Geometry check sheet. Reference: the model listing, model coordinates, mm. Face numbers are marked on the shaded views. A direction names the side the tool comes from. Give positions to 0.01 mm unless a question says otherwise; leave off trailing zeros. Order: outer loops, then holes, each group sorted by start corner. A loop starts at its lowest first (then second) coordinate and runs counter-clockwise, first axis right, second up. Notation, with made-up numbers: M -3,41.25 L 29,41.25 A10 cw 29,58.25 Z; hole C 17.5,73 d8. An arc over 180 degrees is marked long. Answer as CSV lines item,"result". Start each with the question number.
Q1. Go/stop test with flat-tipped pins: pin 1 (6 mm diameter, centred on x = 73.5, z = -8, fed in from -Y); pin 2 (3 mm diameter, centred on y = 19, z = -39.5, fed in from +X); pin 3 (6 mm diameter, centred on y = 28.5, z = -6.5, fed in from -X). Record where each tip stops, or that it passes through.
Q2. Section check C-C, the plane x = 60.5. Record the boundary of the cut face in (y, z) (3 decimals), then the cut area to 3 significant figures.
Q3. Set-up check for the marked faces 1 and 2: record each of +Z, -Z, +X, -X, +Y, -Y from which the full face is reachable in a straight line by a thin tool's end or side.
Q4. Section check B-B, the plane x = 25. Count the separate pieces of the cut face and the enclosed holes in it, then the cut area to 3 significant figures.
Q5. Thickness scan on line 1 (Y direction, x = 25, z = -40.5); line 2 (X direction, y = 10.75, z = -40); line 3 (Z direction, x = 37.5, y = 21.25). Record the ranges inside material, lowest first.
Q6. Mould release check, pull along Z, two halves, no side actions. Record for the marked faces 3, 4 and 5: +Z half, -Z half, draft (parallel to the pull), parting line (faces both ways), or undercut.
Q7. Section check A-A, the plane x = 80. Record the boundary of the cut face in (y, z) (3 decimals), then the cut area to 3 significant figures.
```python
from build123d import *

# Parameters (mm, degrees)
SKETCH_1_W               = 90
SKETCH_1_H               = 45
EXTRUDE_1_DEPTH          = 60
CUT_EXTRUDE_1_DEPTH      = 118.153745139
CUT_EXTRUDE_1_DEPTH_BACK = 118.153745139
CUT_EXTRUDE_2_DEPTH      = 105.446158378
EXTRUDE_3_REACH          = 105.804
SKETCH_4_W               = 86
SKETCH_4_H               = 41
SKETCH_4_W_2             = 82
SKETCH_4_H_2             = 34
CUT_EXTRUDE_3_DEPTH      = 105.522724802
SKETCH_6_W               = 72
SKETCH_6_H               = 33
CUT_EXTRUDE_4_DEPTH      = 98.541192544
EXTRUDE_8_DEPTH          = 82
CUT_EXTRUDE_5_REACH      = 99.614
SKETCH_10_W              = 79
SKETCH_10_H              = 27.766838789
SKETCH_11_W              = 3
SKETCH_11_H              = 42.766838789
CUT_EXTRUDE_6_DEPTH      = 5
EXTRUDE_9_DEPTH          = 28
SKETCH_13_R              = 1.5
CUT_EXTRUDE_7_DEPTH      = 104.169264805
FILLET_1_R               = 1
FILLET_2_R               = 1
FILLET_3_R               = 1
CUT_EXTRUDE_8_DEPTH      = 1


with BuildPart() as part:
    # 草图1 → 凸台-拉伸1 (new body)
    with BuildSketch(Plane(origin=(0, 0, 0), x_dir=(1, 0, 0), z_dir=(0, 1, 0))):
        with Locations((45, 22.5)):
            Rectangle(SKETCH_1_W, SKETCH_1_H)
    extrude(amount=EXTRUDE_1_DEPTH)

    # 草图2 → 切除-拉伸1 (cut, two sides: drawn at the far end of the back side and taken through both)
    with BuildSketch(Plane(origin=(90, 0, 0), x_dir=(0, 0, -1), z_dir=(1, 0, 0)).offset(-CUT_EXTRUDE_1_DEPTH_BACK)):
        Polygon((0, 220), (0, 60), (0, 28), (40, 10), (45, 10), (205, 10), (433.983745882, 233.531751932), (228.983745882, 443.531751932), align=None)
    extrude(amount=CUT_EXTRUDE_1_DEPTH + CUT_EXTRUDE_1_DEPTH_BACK, mode=Mode.SUBTRACT)

    # 草图3 → 切除-拉伸2 (cut, through all)
    with BuildSketch(Plane(origin=(90, 0, 0), x_dir=(0, 0, -1), z_dir=(1, 0, 0))):
        Polygon((0, 26.44865757), (39.885905712, 8.5), (45, 8.5), (45, 0), (0, 0), align=None)
    extrude(amount=-CUT_EXTRUDE_2_DEPTH, mode=Mode.SUBTRACT)

    # 草图4 → 凸台-拉伸3 (add, up to next)
    with BuildSketch(Plane(origin=(0, 34, 0), x_dir=(1, 0, 0), z_dir=(0, 1, 0)), mode=Mode.PRIVATE) as extrude_3_sk1:
        with Locations((45, 22.5)):
            Rectangle(SKETCH_4_W, SKETCH_4_H)
        with Locations((45, 21)):
            Rectangle(SKETCH_4_W_2, SKETCH_4_H_2, mode=Mode.SUBTRACT)
    extrude_3_tool1 = extrude(extrude_3_sk1.sketch, amount=-EXTRUDE_3_REACH, mode=Mode.PRIVATE) - part.part
    add(extrude_3_tool1.solids().sort_by_distance((45, 34, -2.952733))[0])

    # 草图5 → 切除-拉伸3 (cut, through all)
    with BuildSketch(Plane.ZY.offset(-2)):
        Polygon((-43, 15.03292805), (-41, 15.03292805), (-2, 32.58292805), (-2, 34), (-43, 34), align=None)
    extrude(amount=-CUT_EXTRUDE_3_DEPTH, mode=Mode.SUBTRACT)

    # 草图6 → 切除-拉伸4 (cut, through all)
    with BuildSketch(Plane(origin=(0, 21.99472563, -9.897626534), x_dir=(1, 0, 0), z_dir=(0, -0.9119215051751064, 0.41036467732879806))):
        with Locations((49, -11.015560293)):
            Rectangle(SKETCH_6_W, SKETCH_6_H)
    extrude(amount=-CUT_EXTRUDE_4_DEPTH, mode=Mode.SUBTRACT)

    # 草图9 → 凸台-拉伸8 (add)
    with BuildSketch(Plane(origin=(4, 0, 0), x_dir=(0, 0, -1), z_dir=(1, 0, 0))):
        Polygon((4, 31.68292805), (4, 30.58634244), (38, 15.28634244), (38, 16.38292805), align=None)
    extrude(amount=EXTRUDE_8_DEPTH)

    # 草图10 → 切除-拉伸5 (cut, up to next)
    with BuildSketch(Plane(origin=(0, 27.844430811, -12.529993865), x_dir=(1, 0, 0), z_dir=(0, 0.9119215051751064, -0.410364677328798)), mode=Mode.PRIVATE) as cut_extrude_5_sk1:
        with Locations((44.5, 10.33637965)):
            Rectangle(SKETCH_10_W, SKETCH_10_H)
    cut_extrude_5_tool1 = extrude(cut_extrude_5_sk1.sketch, amount=-CUT_EXTRUDE_5_REACH, mode=Mode.PRIVATE) & part.part
    add(cut_extrude_5_tool1.solids().sort_by_distance((44.5, 23.602746, -21.955961))[0], mode=Mode.SUBTRACT)

    # 草图11 → 切除-拉伸6 (cut)
    with BuildSketch(Plane(origin=(0, 27.844430811, -12.529993865), x_dir=(1, 0, 0), z_dir=(0, 0.9119215051751064, -0.410364677328798))):
        with Locations((3.5, 9.836379649)):
            Rectangle(SKETCH_11_W, SKETCH_11_H)
    extrude(amount=-CUT_EXTRUDE_6_DEPTH, mode=Mode.SUBTRACT)

    # 草图12 → 凸台-拉伸9 (add, symmetric)
    with BuildSketch(Plane(origin=(45, 0, 0), x_dir=(0, 0, -1), z_dir=(1, 0, 0))):
        Polygon((43, 15.03292805), (43, 17.095415955), (41.5, 17.095415955), (41.5, 27.095415955), (38.5, 27.095415955), (38.5, 15.06134244), (41, 15.03292805), align=None)
    extrude(amount=EXTRUDE_9_DEPTH, both=True)

    # 草图13 → 切除-拉伸7 (cut, through all)
    with BuildSketch(Plane.XY.offset(-38.5)):
        with Locations((25, 22)):
            Circle(SKETCH_13_R)
        with Locations((65, 22)):
            Circle(SKETCH_13_R)
    extrude(amount=-CUT_EXTRUDE_7_DEPTH, mode=Mode.SUBTRACT)

    # 圆角1
    fillet_1_edges = [part.edges().sort_by_distance(p)[0] for p in [
        (13, 11.348360437, -35.279929664),
        (13, 24.890394788, -5.186519993),
        (85, 24.890394788, -5.186519993),
        (85, 11.348360437, -35.279929664),
        (90, 27.224328785, 0),
        (0, 27.224328785, 0),
        (0, 17.474328785, -19.942952856),
        (45, 26.44865757, 0),
        (0, 8.5, -42.442952856),
        (45, 8.5, -39.885905712),
        (90, 8.5, -42.442952856),
        (90, 17.474328785, -19.942952856),
    ]]
    fillet(fillet_1_edges, radius=FILLET_1_R)

    # 圆角2
    fillet_2_edges = [part.edges().sort_by_distance(p)[0] for p in [
        (45, 16.15792805, -38.5),
        (73, 27.095415955, -40),
        (17, 27.095415955, -40),
    ]]
    fillet(fillet_2_edges, radius=FILLET_2_R)

    # 圆角3
    # the kernel refuses this fillet: 1 mm, written as the material it adds along each edge
    with BuildSketch(Plane(origin=(84, 29.300010631, -9.295372041), x_dir=(0, -0.4103646773287979, -0.9119215051751064), z_dir=(0, -0.9119215051751064, 0.41036467732879794)), Plane(origin=(84, 17.905480791, -34.616549464), x_dir=(-1, 0, 0), z_dir=(0, -0.9119215051751064, 0.41036467732879794))) as fillet_3_piece_1:
        with BuildLine():
            CenterArc((FILLET_3_R, -FILLET_3_R), FILLET_3_R, 90, 90)
            Line((0, -FILLET_3_R), (0, 0))
            Line((0, 0), (FILLET_3_R, 0))
        make_face()
    extrude(amount=1)
    with BuildSketch(Plane(origin=(5, 15.03292805, -41), x_dir=(-1, 0, 0), z_dir=(0, -0.9119215051751064, 0.410364677328798))) as fillet_3_piece_2_section:
        with BuildLine():
            CenterArc((FILLET_3_R, -FILLET_3_R), FILLET_3_R, 90, 90)
            Line((0, -FILLET_3_R), (0, 0))
            Line((0, 0), (FILLET_3_R, 0))
        make_face()
    fillet_3_piece_2 = extrude(amount=7.5, mode=Mode.PRIVATE)
    fillet_3_piece_2 = split(fillet_3_piece_2, bisect_by=Plane(origin=(4.869229562, 9.339477608, -38.020399916), z_dir=(0, 0.9119215051751064, -0.41036467732879794)), keep=Keep.TOP, mode=Mode.PRIVATE)
    add(fillet_3_piece_2)
    # the kernel refuses this fillet: 1 mm, written as the material it takes off along each edge
    with BuildSketch(Plane(origin=(88, 17.53292805, -43), x_dir=(-1, 0, 0), z_dir=(0, -1, 0))) as fillet_3_2_piece_1:
        with BuildLine():
            CenterArc((FILLET_3_R, -FILLET_3_R), FILLET_3_R, 90, 90)
            Line((0, -FILLET_3_R), (0, 0))
            Line((0, 0), (FILLET_3_R, 0))
        make_face()
    extrude(amount=7.53292805, mode=Mode.SUBTRACT)
    with BuildSketch(Plane(origin=(2, 17.53292805, -43), x_dir=(1, 0, 0), z_dir=(0, -1, 0))) as fillet_3_2_piece_2:
        with BuildLine():
            CenterArc((FILLET_3_R, FILLET_3_R), FILLET_3_R, 180, 90)
            Line((0, FILLET_3_R), (0, 0))
            Line((0, 0), (FILLET_3_R, 0))
        make_face()
    extrude(amount=7.53292805, mode=Mode.SUBTRACT)
    with BuildSketch(Plane(origin=(5, 31.579814394, -10.321283735), x_dir=(1, 0, 0), z_dir=(0, -0.9119215051751064, 0.41036467732879794)), Plane(origin=(5, 20.185284554, -35.642461157), x_dir=(0, -0.4103646773287979, -0.9119215051751064), z_dir=(0, -0.9119215051751064, 0.41036467732879794))) as fillet_3_2_piece_3:
        with BuildLine():
            CenterArc((FILLET_3_R, FILLET_3_R), FILLET_3_R, 180, 90)
            Line((0, FILLET_3_R), (0, 0))
            Line((0, 0), (FILLET_3_R, 0))
        make_face()
    extrude(amount=6, mode=Mode.SUBTRACT)
    with BuildSketch(Plane(origin=(2, 17.312731813, -42.025911693), x_dir=(0, -0.410364677328798, -0.9119215051751063), z_dir=(0, -0.9119215051751064, 0.410364677328798))) as fillet_3_2_piece_4:
        with BuildLine():
            CenterArc((FILLET_3_R, FILLET_3_R), FILLET_3_R, 180, 90)
            Line((0, FILLET_3_R), (0, 0))
            Line((0, 0), (FILLET_3_R, 0))
        make_face()
    extrude(amount=7.5, mode=Mode.SUBTRACT)
    with BuildSketch(Plane(origin=(5, 35.08292805, -2), x_dir=(0, 0, -1), z_dir=(0, -1, 0))) as fillet_3_2_piece_5_section:
        with BuildLine():
            CenterArc((FILLET_3_R, FILLET_3_R), FILLET_3_R, 180, 90)
            Line((0, FILLET_3_R), (0, 0))
            Line((0, 0), (FILLET_3_R, 0))
        make_face()
    fillet_3_2_piece_5 = extrude(amount=10.48292805, mode=Mode.PRIVATE)
    fillet_3_2_piece_5 = split(fillet_3_2_piece_5, bisect_by=Plane(origin=(5.223367939, 27.46114469, -1.197456246), z_dir=(0, 0.9119215051751064, -0.4103646773287979)), keep=Keep.TOP, mode=Mode.PRIVATE)
    add(fillet_3_2_piece_5, mode=Mode.SUBTRACT)
    with BuildSketch(Plane(origin=(88, 35.08292805, -2), x_dir=(-1, 0, 0), z_dir=(0, -1, 0))) as fillet_3_2_piece_6_section:
        with BuildLine():
            CenterArc((FILLET_3_R, FILLET_3_R), FILLET_3_R, 180, 90)
            Line((0, FILLET_3_R), (0, 0))
            Line((0, 0), (FILLET_3_R, 0))
        make_face()
    fillet_3_2_piece_6 = extrude(amount=10.48292805, mode=Mode.PRIVATE)
    fillet_3_2_piece_6 = split(fillet_3_2_piece_6, bisect_by=Plane(origin=(87.776632061, 27.46114469, -1.197456246), z_dir=(0, 0.9119215051751064, -0.4103646773287979)), keep=Keep.TOP, mode=Mode.PRIVATE)
    add(fillet_3_2_piece_6, mode=Mode.SUBTRACT)

    # 草图14 → 切除-拉伸8 (cut)
    with BuildSketch(Plane(origin=(0, 21.99472563, -9.897626534), x_dir=(1, 0, 0), z_dir=(0, -0.9119215051751063, 0.4103646773287981))):
        with BuildLine():
            Line((9, 3.984439707), (9, -26.015560293))
            ThreePointArc((9, -26.015560293), (8, -27.015560293), (7, -26.015560293))
            Line((7, -26.015560293), (7, 3.984439707))
            ThreePointArc((7, 3.984439707), (8, 4.984439707), (9, 3.984439707))
        make_face()
        with BuildLine():
            Line((3, -1.015560293), (3, 3.984439707))
            ThreePointArc((3, 3.984439707), (4, 4.984439707), (5, 3.984439707))
            Line((5, 3.984439707), (5, -1.015560293))
            ThreePointArc((5, -1.015560293), (4, -2.015560293), (3, -1.015560293))
        make_face()
    extrude(amount=-CUT_EXTRUDE_8_DEPTH, mode=Mode.SUBTRACT)


solid = part.part
```
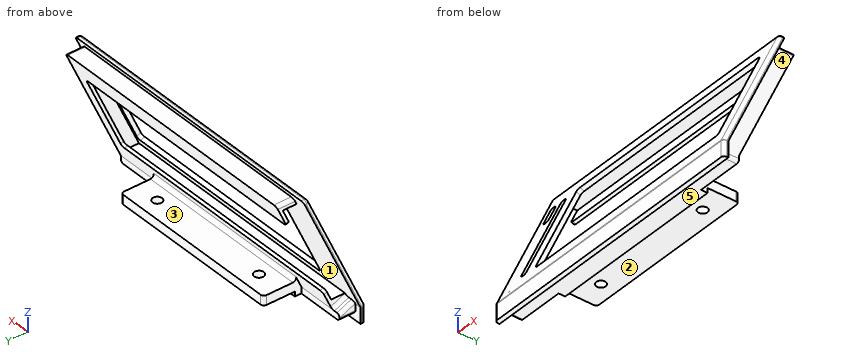
Answer block:
1,pin 1,"stops at y = 24.48"
1,pin 2,"stops at x = 73"
1,pin 3,"stops at x = 5"
2,outline,"M 8.5,-45 L 10,-45 L 10,-43 L 17.095,-43 L 17.095,-41.5 L 27.095,-41.5 L 27.095,-38.5 L 17.705,-38.5 A1 cw 16.793,-37.09 L 17.905,-34.617 L 16.994,-34.206 L 15.286,-38 L 10.9,-38 L 11.993,-35.57 L 10.703,-34.99 L 8.588,-39.69 A1 ccw 8.5,-40.101 Z; M 24.245,-4.896 L 25.535,-5.477 L 26.2,-4 L 30.586,-4 L 28.388,-8.885 L 29.3,-9.295 L 32.583,-2 L 27.1,-2 L 28,0 L 27.095,0 A1 ccw 26.183,-0.59 Z"
2,area,"108 mm2"
3,face 1,"none"
3,face 2,"-Z, +X, -X, +Y"
4,separate pieces,"3"
4,enclosed holes,"0"
4,area,"99.0 mm2"
5,line 1,"y = 8.5 to 20.5, 23.5 to 27.1"
5,line 2,"x = 2.01 to 88"
5,line 3,"z = -41.5 to -38.5"
6,face 3,"undercut"
6,face 4,"draft"
6,face 5,"-Z half"
7,outline,"M 8.5,-45 L 10,-45 L 10,-43 L 15.033,-43 L 15.033,-41 L 17.905,-34.617 L 16.994,-34.206 L 15.286,-38 L 10.9,-38 L 11.993,-35.57 L 10.703,-34.99 L 8.588,-39.69 A1 ccw 8.5,-40.101 Z; M 24.245,-4.896 L 25.535,-5.477 L 26.2,-4 L 30.586,-4 L 28.388,-8.885 L 29.3,-9.295 L 32.583,-2 L 27.1,-2 L 28,0 L 27.095,0 A1 ccw 26.183,-0.59 Z"
7,area,"69.6 mm2"
